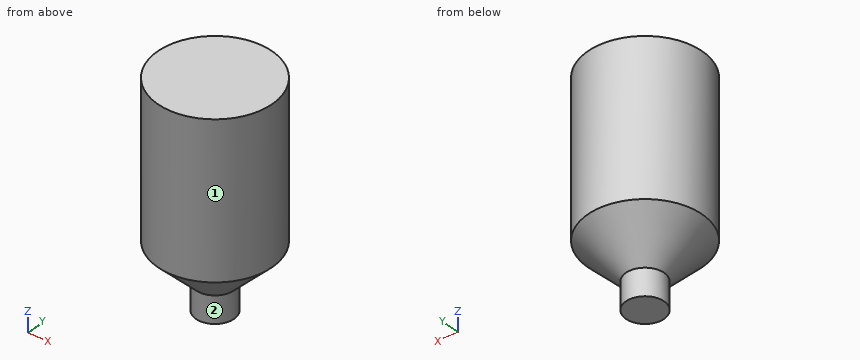
from build123d import *

# Parameters (mm, degrees)
F0_R     = 38.1
F1_DEPTH = 101.6
F2_R     = 38.1
F3_DEPTH = 25.4
F3_TAPER = 45
F4_R     = 12.7
F5_DEPTH = 17.78


with BuildPart() as f1:
    # F0 (on Top) → F1 (new body)
    with BuildSketch(Plane.XY):
        Circle(F0_R)
    extrude(amount=-F1_DEPTH)

    # F2 (on face) → F3 (join)
    with BuildSketch(Plane(origin=(0, 0, -101.6), x_dir=(1, 0, 0), z_dir=(0, 0, -1))):
        Circle(F2_R)
    extrude(amount=F3_DEPTH, taper=F3_TAPER)

    # F4 (on face) → F5 (join)
    with BuildSketch(Plane(origin=(0, 0, -127), x_dir=(1, 0, 0), z_dir=(0, 0, -1))):
        Circle(F4_R)
    extrude(amount=F5_DEPTH)


solid = f1.part
Check sheet for the modelled part. Datum: model origin and axes. Units: mm. Face numbers are marked on the shaded views. A direction names the side the tool comes from. Coordinates: 2 decimals unless noted, no trailing zeros. Write each loop counter-clockwise with the first axis right and the second up, starting at its lowest first coordinate (ties: lowest second). Pieces come first, ordered by that corner, then holes.
Item 1: Cross-section at C-C on z = -74. Record the boundary of the cut face in (x, y), then the cut area to 3 significant figures.
Numbers:
outline: circle Ø76.2 at (0, 0)
area: 4,560 mm2
Item 2: Cross-section at A-A on x = 0. Record the boundary of the cut face in (y, z).
Numbers:
outline: (-38.1, -101.6) - (-12.7, -127) - (-12.7, -144.78) - (12.7, -144.78) - (12.7, -127) - (38.1, -101.6) - (38.1, 0) - (-38.1, 0) - close
Item 3: Depth check by flat-ended pin: pin 1 Ø6 at (x, z) = (-13.5, -83) entering from -Y; pin 2 Ø10 at (x, z) = (-2.5, -28.5) entering from -Y; pin 3 Ø5 at (y, z) = (5.5, -103) entering from -X. Enter the tip coordinate at first touch or a pass-through.
Numbers:
pin 1: stops at y = -36.62
pin 2: stops at y = -38.1
pin 3: stops at x = -37.95
Item 4: Access from +Z, -Z, +X, -X, +Y, -Y to the whole of each face (thin tool, end or side, straight path). Record for the marked faces 1 and 2.
Numbers:
face 1: +Z, -Z
face 2: -Z
Item 5: Scan lines: probe 1 along Y at (x, z) = (-1, -40.5); probe 2 along Y at (x, z) = (-26.5, -15). Record each from-to range of solid material in increasing order.
Numbers:
probe 1: y = -38.09 to 38.09
probe 2: y = -27.37 to 27.37
Item 6: Cross-section at B-B on z = -109. Record the boundary of the cut face in (x, y).
Numbers:
outline: circle Ø61.4 at (0, 0)
